Build history of the part. All positions in model axes, mm. Face numbers are marked on the shaded views. Give positions to 0.01 mm unless a question says otherwise; leave off trailing zeros. Write each loop counter-clockwise with the first axis right and the second up, starting at its lowest first coordinate (ties: lowest second). Pieces come first, ordered by that corner, then holes.
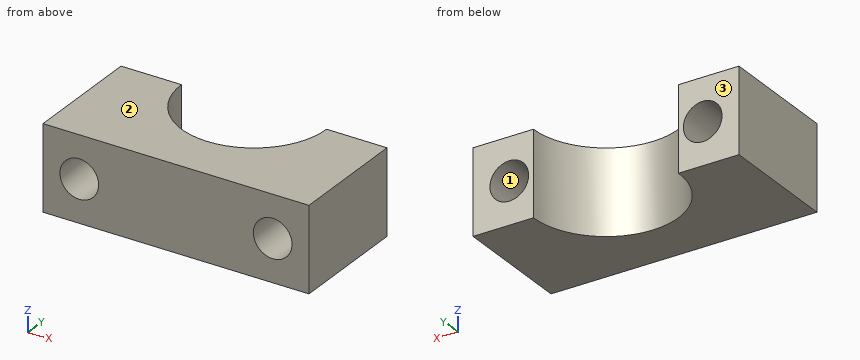
Autodesk Inventor part; units mm, degrees
ref_plane "YZ Plane" through (0, 0, 0) normal (1, 0, 0) x (0, 1, 0)
ref_plane "XZ Plane" through (0, 0, 0) normal (0, 1, 0) x (-1, 0, 0)
ref_plane "XY Plane" through (0, 0, 0) normal (0, 0, 1) x (1, 0, 0)
sketch "Sketch2" plane through (0, 0, 0) normal (0, 0, 1) x (1, 0, 0)
  circle A0 centre (0, 0) radius 6
  line L0 (-11, 0) -> (11, 0)
  line L1 (11, 0) -> (11, -10)
  line L2 (11, -10) -> (-11, -10)
  line L3 (-11, -10) -> (-11, 0)
  circle A1 centre (0, 0) radius 9
  point P0 (6, 0)
  point P1 (-6, 0)
  dimension "d0" = 12
  dimension "d1" = 11
  dimension "d2" = 11
  dimension "d3" = 10
  dimension "d4" = 3
extrude "Extrusion1" add sketch "Sketch2" along normal blind 7 contours L0 A1 A0 | L0 L1 L2 L3 A1 picked at (-7.9128, -0.7179)
sketch "Sketch3" plane through (6, 0, 0) normal (0, 1, 0) x (1, 0, 0)
  circle A0 centre (2, -3.5) radius 1.6
  line L0 (5, 0) -> (5, -7)
  line L1 (5, 0) -> (0, 0)
  circle A1 centre (-14, -3.5) radius 1.6
  line L2 (-17, 0) -> (-17, -7)
  line L3 (-12, 0) -> (-17, 0)
  point P0 (-6, 0)
  dimension "d7" = 3.2
  dimension "d8" = 3
  dimension "d9" = 3.5
  dimension "d10" = 3.2
  dimension "d11" = 3
  dimension "d12" = 3.5
extrude "Extrusion2" cut sketch "Sketch3" against normal blind 10
properties part number "Tube_mount"
(1) Drop a flat-ended pin along its axis: pin 1 (2.5 mm diameter, centred on x = 8, z = 3.5, fed in from -Y). Give the stop position or say it passes through.
(2) Mould opens along Z. For the marked faces 1, 2 and 3 say: +Z half, -Z half, draft (parallel to the pull), parting line (faces both ways), or undercut.
(3) Saw through at B-B, the plane z = 3.5. List the corners of the cut face in (x, y), plus the area to 3 significant figures.
(4) Saw through at A-A, the plane x = 8. List the corners of the cut face in (y, z).
(5) Probe line 1 (X direction, y = -8, z = 3.5); line 2 (Z direction, x = -8, y = -3.5); line 3 (X direction, y = -7, z = 4). List the from-to ranges inside material, lowest first.
(6) Saw through at C-C, the plane y = -5. List the corners of the cut face in (x, z).
(7) Saw through at D-D, the plane y = -9.5. List the corners of the cut face in (x, z).
Computed values:
1. pin 1: passes through
2. face 1: undercut
2. face 2: +Z half
2. face 3: draft
3. outline: (-11, -10) - (-9.6, -10) - (-9.6, 0) - (-11, 0) - close; (-6.4, -10) - (6.4, -10) - (6.4, 0) - (6, 0) arc R6 cw to (-6, 0) - (-6.4, 0) - close; (9.6, -10) - (11, -10) - (11, 0) - (9.6, 0) - close
3. area: 99.5 mm2
4. outline: (-10, 0) - (0, 0) - (0, 1.9) - (-10, 1.9) - close; (-10, 5.1) - (0, 5.1) - (0, 7) - (-10, 7) - close
5. line 1: x = -11 to -9.6, -6.4 to 6.4, 9.6 to 11
5. line 2: z = 0 to 1.9, 5.1 to 7
5. line 3: x = -11 to -9.52, -6.48 to 6.48, 9.52 to 11
6. outline: (-11, 0) - (-3.32, 0) - (-3.32, 7) - (-11, 7) - close; (3.32, 0) - (11, 0) - (11, 7) - (3.32, 7) - close; hole circle Ø3.2 at (-8, 3.5); hole circle Ø3.2 at (8, 3.5)
7. outline: (-11, 0) - (11, 0) - (11, 7) - (-11, 7) - close; hole circle Ø3.2 at (-8, 3.5); hole circle Ø3.2 at (8, 3.5)
